Geometry: see drawing. Coordinates: mm, zero at the bounding-box minimum. Round coordinates to 2 decimals unless told otherwise and drop trailing zeros. Order: outer loops, then holes, each group sorted by start corner. A loop starts at its lowest first (then second) coordinate and runs counter-clockwise, first axis right, second up. Notation, with made-up numbers: (14.5, 20.25) -> (46.5, 20.25) arc R21 cw to (46.5, 51.25) -> close; hole circle Ø4 at (86, 48.5). An arc over 180 degrees is marked (long way). One line per item, written item: value. Start each with the question number.
1) Ray query, L1, parallel to X at y = 12, z = 3 (1 decimal); L2, parallel to Z at x = 2.9, y = 9; L3, parallel to Z at x = 3.5, y = 7 (1 decimal). Return the intervals inside material, ascending.
2) Section B-B (y = 8.75). Return the cut outline in (x, z) (1 decimal).
3) Mould query, pull axis X, two halves, no side actions, for the marked faces 1 and 2. Classes: pulls with the +X half, pulls with the -X half, needs draft (parallel to the pull), parting line crosses it, or undercut.
4) Pin query (flat end, axial travel): P1, Ø0.5, axis at x = 0.5, y = 5.5, coming from the +Z side; P2, Ø0.8, axis at x = 0.5, y = 13, coming from the -Z side; P3, Ø2, axis at y = 5.5, z = 4.5, coming from the -X side. Return the tip coordinate at first contact, or that it passes through.
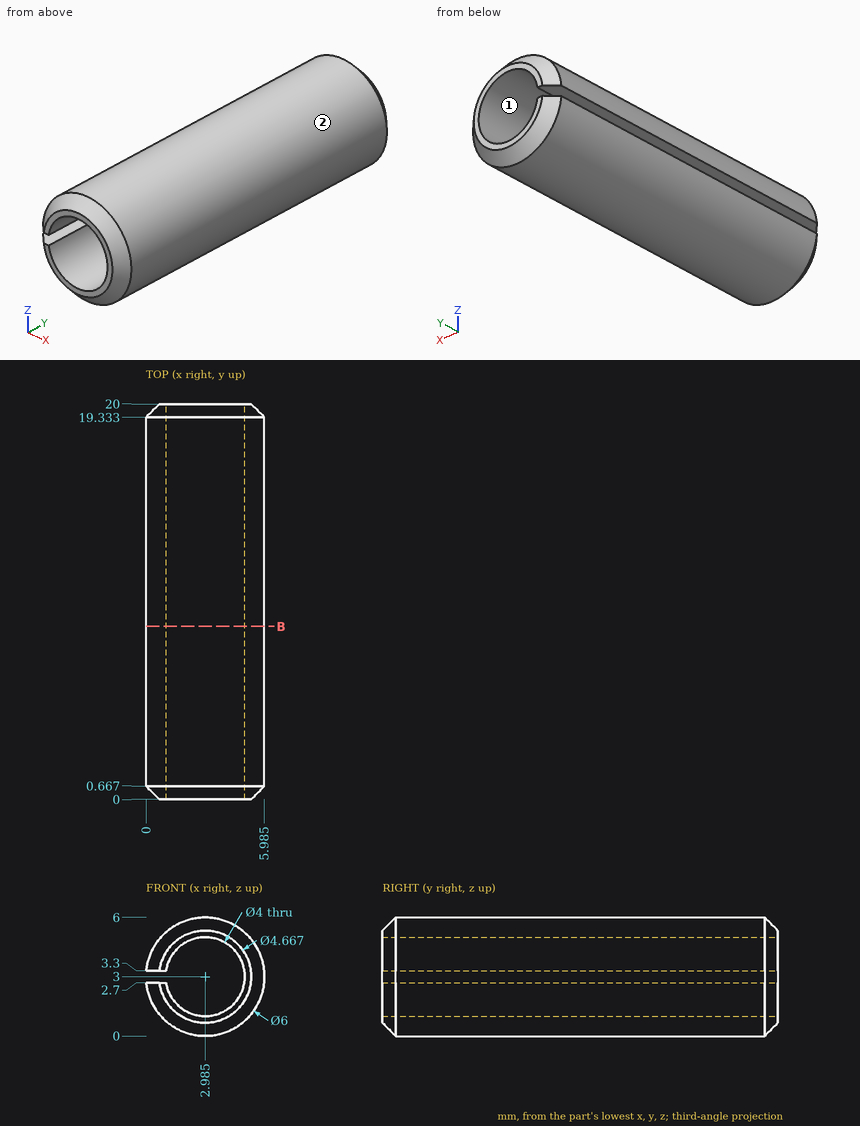
Findings:
1. L1: 5 to 6
1. L2: 0 to 1, 5 to 6
1. L3: 0 to 1.1, 4.9 to 6
2. outline: (0, 2.7) arc R3 ccw (long way) to (0, 3.3) -> (1, 3.3) arc R2 cw (long way) to (1, 2.7) -> close
3. face 1: undercut
3. face 2: parting line crosses it
4. P1: z = 5
4. P2: z = 0.84
4. P3: x = 0.03
